For this review, take the finished solid that the model builds, in its own axes (mm). A direction names the side the tool comes from. Coordinates: 2 decimals unless noted, no trailing zeros. Write each loop counter-clockwise with the first axis right and the second up, starting at its lowest first coordinate (ties: lowest second). Pieces come first, ordered by that corner, then holes. Notation, with made-up numbers: M 64,42.25 L 75,42.25 A8 cw 75,47.25 Z; hole C -40,36.25 d7. An arc over 180 degrees is marked long. One line per question, with ' | ' between items.
from build123d import *

# Parameters (mm, degrees)
BASE_FLANGE1_DEPTH = 35
CUT_EXTRUDE1_REACH = 79.942
CUT_EXTRUDE2_REACH = 79.942
SKETCH7_R          = 4
CUT_EXTRUDE3_REACH = 77.492
SKETCH8_R          = 3.75
CHAMFER1_SIZE      = 2.5


# Sheet-metal steps are written as plain solids
with BuildPart() as part:
    # Sketch1 → Base-Flange1 (new body)
    with BuildSketch(Plane.XY):
        with BuildLine():
            Line((0, 0), (0, -33))
            ThreePointArc((0, -33), (0.585786438, -34.414213562), (2, -35))
            Line((2, -35), (53, -35))
            ThreePointArc((53, -35), (54.414213562, -34.414213562), (55, -33))
            Line((55, -33), (55, 0))
            Line((55, 0), (57, 0))
            Line((57, 0), (57, -33))
            ThreePointArc((57, -33), (55.828427125, -35.828427125), (53, -37))
            Line((53, -37), (2, -37))
            ThreePointArc((2, -37), (-0.828427125, -35.828427125), (-2, -33))
            Line((-2, -33), (-2, 0))
            Line((-2, 0), (0, 0))
        make_face()
    extrude(amount=BASE_FLANGE1_DEPTH)

    # Sketch6 → Cut-Extrude1 (cut, up to next)
    with BuildSketch(Plane(origin=(57, 0, 0), x_dir=(0, 0, -1), z_dir=(1, 0, 0)), mode=Mode.PRIVATE) as cut_extrude1_sk1:
        with BuildLine():
            ThreePointArc((-18.525, -8.545539774), (-30, -11), (-18.525, -13.454460226))
            ThreePointArc((-18.525, -13.454460226), (-16.5, -11), (-18.525, -8.545539774))
        make_face()
    cut_extrude1_tool1 = extrude(cut_extrude1_sk1.sketch, amount=-CUT_EXTRUDE1_REACH, mode=Mode.PRIVATE) & part.part
    add(cut_extrude1_tool1.solids().sort_by_distance((57, -11, 23.686214))[0], mode=Mode.SUBTRACT)

    # Sketch7 → Cut-Extrude2 (cut, up to next)
    with BuildSketch(Plane.ZY.offset(2), mode=Mode.PRIVATE) as cut_extrude2_sk1:
        with Locations((24, -11)):
            Circle(SKETCH7_R)
    cut_extrude2_tool1 = extrude(cut_extrude2_sk1.sketch, amount=-CUT_EXTRUDE2_REACH, mode=Mode.PRIVATE) & part.part
    add(cut_extrude2_tool1.solids().sort_by_distance((-2, -11, 24))[0], mode=Mode.SUBTRACT)

    # Sketch8 → Cut-Extrude3 (cut, up to next)
    with BuildSketch(Plane(origin=(0, -35, 0), x_dir=(1, 0, 0), z_dir=(0, 1, 0)), mode=Mode.PRIVATE) as cut_extrude3_sk1:
        with Locations(Location((27.5, -17.5, 0), (0, 0, 270))):
            Circle(SKETCH8_R)
    cut_extrude3_tool1 = extrude(cut_extrude3_sk1.sketch, amount=-CUT_EXTRUDE3_REACH, mode=Mode.PRIVATE) & part.part
    add(cut_extrude3_tool1.solids().sort_by_distance((27.5, -35, 17.5))[0], mode=Mode.SUBTRACT)

    # Chamfer1
    chamfer1_edges = [part.edges().sort_by_distance(p)[0] for p in [
        (-1, 0, 0),
        (56, 0, 0),
        (-1, 0, 35),
        (56, 0, 35),
    ]]
    chamfer(chamfer1_edges, length=CHAMFER1_SIZE)


solid = part.part
1) We need section C-C on z = 17.5. State the section outline as (x, y) points.
Responses:
outline: M -2,-33 A4 ccw 2,-37 L 23.75,-37 L 23.75,-35 L 2,-35 A2 cw 0,-33 L 0,0 L -2,0 Z; M 31.25,-37 L 53,-37 A4 ccw 57,-33 L 57,-13 L 55,-13 L 55,-33 A2 cw 53,-35 L 31.25,-35 Z; M 55,-9 L 57,-9 L 57,0 L 55,0 Z
2) We need section D-D on y = -11. State the section outline as (x, z) points.
Responses:
outline: M -2,0 L 0,0 L 0,20 L -2,20 Z; M -2,28 L 0,28 L 0,35 L -2,35 Z; M 55,0 L 57,0 L 57,16.5 L 55,16.5 Z; M 55,30 L 57,30 L 57,35 L 55,35 Z
3) The part is to be moulded in two halves that separate along Z. For faces 1 (the flat face through (-1, 0, 17)), 2 (the cylindrical face through (56, -11, 30)), 3 (the cylindrical face through (27.665, -35.986, 13.754)), 4 (the flat face through (56, -1.2, 1.3)), say which applies: +Z half, -Z half, draft (parallel to the pull), parting line (faces both ways), or undercut.
Responses:
face 1: draft | face 2: undercut | face 3: undercut | face 4: -Z half
4) To check wall thickness, follow line 1 along X through (y, z) = (-29, 22.5); line 2 along Z through (x, y) = (56.35, -11); line 3 along X through (y, z) = (-15, 26). State the ranges of each line that lie inside material, in increasing order. Write a range as [from, to].
Responses:
line 1: [-2, 0], [55, 57] | line 2: [0, 16.5], [30, 35] | line 3: [-2, 0]
5) We need section B-B on x = 27.5. State the section outline as (y, z) points, then the cut area to 3 significant figures.
Responses:
outline: M -37,0 L -35,0 L -35,13.75 L -37,13.75 Z; M -37,21.25 L -35,21.25 L -35,35 L -37,35 Z | area: 55.0 mm^2
6) Insertion check: pin 1 Ø9 at (y, z) = (-11, 24) entering from +X; pin 2 Ø6 at (x, z) = (8, 12.5) entering from +Y. Each pin has a flat end and moves straight along its axis. Give the tip position at first contact, or say it passes through.
Responses:
pin 1: x = 0 | pin 2: y = -35
7) Machinability: for faces 5 (the flat face through (55, -17, 17)), 6 (the flat face through (-1, -1.3, 1.2)), 7 (the cylindrical face through (56, -11, 16.5)), which of the approach directions +Z, -Z, +X, -X, +Y, -Y give a long, thin tool a straight path to every point of the face, cutting with its end or side? Answer none if there is none.
Responses:
face 5: +Z, -Z, +Y | face 6: -Z, +X, -X, +Y | face 7: +X
8) We need section A-A on y = -3.5. State the section outline as (x, z) points.
Responses:
outline: M -2,0 L 0,0 L 0,35 L -2,35 Z; M 55,0 L 57,0 L 57,35 L 55,35 Z
